```python
from build123d import *

# Parameters (mm, degrees)
F1_DEPTH = 25
F0_W     = 8
F0_H     = 8
F2_DEPTH = 1
F3_R     = 2.3
F4_DEPTH = 25


with BuildPart() as f1:
    # F0 (on Top) → F1 (new body)
    with BuildSketch(Plane.XY):
        Polygon((42, 23), (-42, 23), (-42, 15), (-50, 15), (-50, -15), (-42, -15), (-42, -23), (42, -23), (42, -15), (50, -15), (50, 15), (42, 15), align=None)
    extrude(amount=F1_DEPTH)

    # F0 (on Top) → F2 (join)
    with BuildSketch(Plane.XY):
        with Locations((-46, -19)):
            Rectangle(F0_W, F0_H)
        with Locations((-46, 19)):
            Rectangle(F0_W, F0_H)
        with Locations((46, 19)):
            Rectangle(F0_W, F0_H)
        with Locations((46, -19)):
            Rectangle(F0_W, F0_H)
        Polygon((42, 23), (-42, 23), (-42, 15), (-50, 15), (-50, -15), (-42, -15), (-42, -23), (42, -23), (42, -15), (50, -15), (50, 15), (42, 15), align=None)
    extrude(amount=-F2_DEPTH)

    # F3 (on Top) → F4 (cut)
    with BuildSketch(Plane.XY):
        with Locations((-46.5, -19.1)):
            Circle(F3_R)
        with Locations((46.5, -19.1)):
            Circle(F3_R)
        with Locations((-46.5, 19.1)):
            Circle(F3_R)
        with Locations((46.5, 19.1)):
            Circle(F3_R)
    extrude(amount=-F4_DEPTH, mode=Mode.SUBTRACT)


solid = f1.part
```
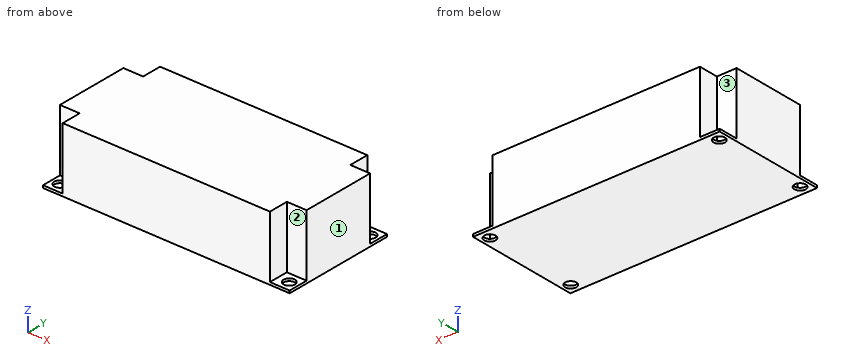
The listing builds one solid part. Answer for the finished solid, in the listing's coordinates (mm). Face numbers are marked on the shaded views. A direction names the side the tool comes from. Coordinates: 2 decimals unless noted, no trailing zeros. Write each loop counter-clockwise with the first axis right and the second up, starting at its lowest first coordinate (ties: lowest second). Pieces come first, ordered by that corner, then holes. Notation, with made-up numbers: M 52,68 L 87,68 A17 cw 87,79 Z; hole C -39.5,34.5 d5. An arc over 180 degrees is marked long. Use a Markdown table: item, result. Add a question column.
1. Which of the six approach directions +Z, -Z, +X, -X, +Y, -Y give full straight-line access (tool end or side, diameter ignored) to the marked faces 1, 2 and 3?
2. Given P1, Ø4, axis at x = 45.5, y = 20.5, coming from the +Z side; P2, Ø1.5, axis at y = 15.5, z = 18.5, coming from the -X side; P3, Ø3.5, axis at x = -46.5, y = -19.1, coming from the -Z side; P4, Ø2.5, axis at x = -47.5, z = 15, coming from the +Y side, each flat-ended and moving along its own axis, determine where each tip first touches the part or whether it passes through.
3. Section A-A (y = -19.1) is taken. Give the vertices of the cut face in (x, z).
4. Section C-C (z = 21.5) is taken. Give the vertices of the cut face in (x, y), plus the area to 3 significant figures.
5. Section B-B (x = 46.5) is taken. Give the vertices of the cut face in (y, z), plus the area to 3 significant figures.
6. Straight lines are drawn through the part: line 1 along Y through (x, z) = (46.5, -0.5); line 2 along X through (y, z) = (19, 5); line 3 along Z through (x, y) = (44, 18.5). For each, find the intervals that lie inside material, in ascending order. Write a range as [from, to].
Data:
| question | item | result |
|---|---|---|
| 1 | face 1 | +Z, -Z, +X, +Y, -Y |
| 1 | face 2 | +Z, +X, -Y |
| 1 | face 3 | +Z, -X, +Y |
| 2 | P1 | stops at z = 0 |
| 2 | P2 | stops at x = -50 |
| 2 | P3 | passes through |
| 2 | P4 | stops at y = 15 |
| 3 | outline | M -50,-1 L -48.8,-1 L -48.8,0 L -50,0 Z; M -44.2,-1 L 44.2,-1 L 44.2,0 L 42,0 L 42,25 L -42,25 L -42,0 L -44.2,0 Z; M 48.8,-1 L 50,-1 L 50,0 L 48.8,0 Z |
| 4 | outline | M -50,-15 L -42,-15 L -42,-23 L 42,-23 L 42,-15 L 50,-15 L 50,15 L 42,15 L 42,23 L -42,23 L -42,15 L -50,15 Z |
| 4 | area | 4,340 mm2 |
| 5 | outline | M -23,-1 L -21.4,-1 L -21.4,0 L -23,0 Z; M -16.8,-1 L 16.8,-1 L 16.8,0 L 15,0 L 15,25 L -15,25 L -15,0 L -16.8,0 Z; M 21.4,-1 L 23,-1 L 23,0 L 21.4,0 Z |
| 5 | area | 787 mm2 |
| 6 | line 1 | y = [-23, -21.4], [-16.8, 16.8], [21.4, 23] |
| 6 | line 2 | x = [-42, 42] |
| 6 | line 3 | z = [-1, 0] |
